Verification items for the finished model (mm, model axes). A direction names the side the tool comes from. Give positions to 0.01 mm unless a question says otherwise; leave off trailing zeros. Loops run counter-clockwise (first coordinate to the right, second up) from the corner with the lowest first, then second, coordinate; pieces in that order, holes last. Notation, with made-up numbers: M 82.5,88 L 93.5,88 A10 ccw 93.5,94 Z; hole C 78,-32.75 d9. An arc over 180 degrees is marked long. Answer in a Markdown table with one row per item.
```python
from build123d import *

# Parameters (mm, degrees)
F0_W     = 406.4
F0_H     = 609.6
F1_DEPTH = 419.1
F2_R     = 50.8
F4_DEPTH = 381


with BuildPart() as f1:
    # F0 (on Top) → F1 (new body)
    with BuildSketch(Plane.XY):
        Rectangle(F0_W, F0_H)
    extrude(amount=F1_DEPTH)

    # F2
    f2_edges = [f1.edges().sort_by_distance(p)[0] for p in [
        (-203.2, 304.8, 209.55),
        (203.2, 304.8, 209.55),
        (-203.2, -304.8, 209.55),
        (203.2, -304.8, 209.55),
    ]]
    fillet(f2_edges, radius=F2_R)

    # F3 (on face) → F4 (cut)
    with BuildSketch(Plane(origin=(0, 0, 0), x_dir=(1, 0, 0), z_dir=(0, 0, -1))):
        with BuildLine():
            ThreePointArc((152.4, -304.8), (188.3210244843, -289.9210244843), (203.2, -254))
            Line((203.2, -254), (203.2, 254))
            ThreePointArc((203.2, 254), (188.3210244843, 289.9210244843), (152.4, 304.8))
            Line((152.4, 304.8), (-152.4, 304.8))
            ThreePointArc((-152.4, 304.8), (-188.3210244843, 289.9210244843), (-203.2, 254))
            Line((-203.2, 254), (-203.2, -254))
            ThreePointArc((-203.2, -254), (-188.3210244843, -289.9210244843), (-152.4, -304.8))
            Line((-152.4, -304.8), (152.4, -304.8))
        make_face()
        with BuildLine():
            Line((-127, 254), (127, 254))
            ThreePointArc((127, 254), (144.9605122421, 246.5605122421), (152.4, 228.6))
            Line((152.4, 228.6), (152.4, -228.6))
            ThreePointArc((152.4, -228.6), (144.9605122421, -246.5605122421), (127, -254))
            Line((127, -254), (-127, -254))
            ThreePointArc((-127, -254), (-144.9605122421, -246.5605122421), (-152.4, -228.6))
            Line((-152.4, -228.6), (-152.4, 228.6))
            ThreePointArc((-152.4, 228.6), (-144.9605122421, 246.5605122421), (-127, 254))
        make_face(mode=Mode.SUBTRACT)
    extrude(amount=-F4_DEPTH, mode=Mode.SUBTRACT)


solid = f1.part
```
Item 1: Go/stop test with flat-tipped pins: pin 1 (8 mm diameter, centred on x = -42.5, z = 142, fed in from +Y); pin 2 (3 mm diameter, centred on x = 144.5, y = -208, fed in from -Z); pin 3 (12 mm diameter, centred on y = 133, z = 233, fed in from -X). Record where each tip stops, or that it passes through.
Reported:
| item | result |
|---|---|
| pin 1 | stops at y = 254 |
| pin 2 | stops at z = 0 |
| pin 3 | stops at x = -152.4 |
Item 2: Scan lines: L1, parallel to Y at x = 25, z = 127; L2, parallel to X at y = 145, z = 35; L3, parallel to Z at x = -155.5, y = 279.5. Record each from-to range of solid material in increasing order. Write a range as [from, to].
Reported:
| item | result |
|---|---|
| L1 | y = [-254, 254] |
| L2 | x = [-152.4, 152.4] |
| L3 | z = [381, 419.1] |
Item 3: Tool access check on faces 1 (the flat face through (2, 254, 188)), 2 (the flat face through (178, -4, 381)), 3 (the flat face through (-152.4, 3, 188)), 4 (the cylindrical face through (-144.76, 246.76, 187.83)). Record the directions out of +Z, -Z, +X, -X, +Y, -Y that give a thin tool (end or side, any length) a straight path to the whole face; none if there is none.
Reported:
| item | result |
|---|---|
| face 1 | -Z, +X, -X, +Y |
| face 2 | -Z |
| face 3 | -Z, -X, +Y, -Y |
| face 4 | -Z, -X, +Y |
Item 4: Sectioned sample at A-A (z = 311.5). Record the cut outline in (x, y), and give its area (3 significant figures).
Reported:
| item | result |
|---|---|
| outline | M -152.4,-228.6 A25.4 ccw -127,-254 L 127,-254 A25.4 ccw 152.4,-228.6 L 152.4,228.6 A25.4 ccw 127,254 L -127,254 A25.4 ccw -152.4,228.6 Z |
| area | 154,000 mm^2 |
Item 5: Sectioned sample at C-C (x = -162). Record the cut outline in (y, z), and give its area (3 significant figures).
Reported:
| item | result |
|---|---|
| outline | M -303.88,381 L 303.88,381 L 303.88,419.1 L -303.88,419.1 Z |
| area | 23,200 mm^2 |
Item 6: Sectioned sample at B-B (y = 84). Record the cut outline in (x, z), and give its area (3 significant figures).
Reported:
| item | result |
|---|---|
| outline | M -203.2,381 L -152.4,381 L -152.4,0 L 152.4,0 L 152.4,381 L 203.2,381 L 203.2,419.1 L -203.2,419.1 Z |
| area | 132,000 mm^2 |
